from build123d import *

# Parameters (mm, degrees)
F0_W     = 117
F0_H     = 37
F1_DEPTH = 1300
F3_DEPTH = 1300


with BuildPart() as f1:
    # F0 (on Top) → F1 (new body)
    with BuildSketch(Plane.XY):
        with BuildLine():
            ThreePointArc((60, 19.6), (59.882843, 19.882843), (59.6, 20))
            Line((59.6, 20), (-59.6, 20))
            ThreePointArc((-59.6, 20), (-59.882843, 19.882843), (-60, 19.6))
            Line((-60, 19.6), (-60, -19.6))
            ThreePointArc((-60, -19.6), (-59.882843, -19.882843), (-59.6, -20))
            Line((-59.6, -20), (59.6, -20))
            ThreePointArc((59.6, -20), (59.882843, -19.882843), (60, -19.6))
            Line((60, -19.6), (60, 19.6))
        make_face()
        Rectangle(F0_W, F0_H, mode=Mode.SUBTRACT)
    extrude(amount=F1_DEPTH)

    # F2 (on face) → F3 (cut)
    with BuildSketch(Plane.XY.offset(1300)):
        with BuildLine():
            Line((-60, 0), (-58.5, 0))
            Line((-58.5, 0), (-58.5, 18.5))
            Line((-58.5, 18.5), (58.5, 18.5))
            Line((58.5, 18.5), (58.5, 0))
            Line((58.5, 0), (60, 0))
            Line((60, 0), (60, 19.6))
            ThreePointArc((60, 19.6), (59.882843, 19.882843), (59.6, 20))
            Line((59.6, 20), (-59.6, 20))
            ThreePointArc((-59.6, 20), (-59.882843, 19.882843), (-60, 19.6))
            Line((-60, 19.6), (-60, 0))
        make_face()
    extrude(amount=-F3_DEPTH, mode=Mode.SUBTRACT)


solid = f1.part
CAD build for the part. Positions are in the model's coordinates, mm. Round coordinates to 2 decimals unless told otherwise and drop trailing zeros. Loops run counter-clockwise (first coordinate to the right, second up) from the corner with the lowest first, then second, coordinate; pieces in that order, holes last. Notation, with made-up numbers: M 80.25,-24.5 L 107.25,-24.5 A25 ccw 107.25,-1.5 Z; hole C 86,70.5 d8. An arc over 180 degrees is marked long. One line per question, with ' | ' between items. Start each with the question number.
Item 1: Cut at B-B, the plane z = 82. Write the cut outline in (x, y).
Item 2: Two-plate mould, pull along X, no slides. Class faces 1 (the flat face through (-1, -18.5, 641)), 2 (the flat face through (-0.3, -19.6, 1300)), 3 (the flat face through (-60, -10, 641)): pulls with the +X half, pulls with the -X half, needs draft (parallel to the pull), parting line crosses it, or undercut.
Item 3: Wall check: line 1 (X direction, y = -6.5, z = 940); line 2 (Y direction, x = 38, z = 104). Give the ranges that are in metal, low to high.
Item 4: Cut at A-A, the plane y = -13.25. Write the cut outline in (x, z), plus the area to 3 significant figures.
Item 5: Cut at C-C, the plane x = -45.5. Write the cut outline in (y, z).
Item 6: Pin check, flat tip, straight feed: pin 1 Ø12 at (x, z) = (5, 794.5) entering from +Y. Stop position of the tip, or through.
Responses:
1) outline: M -60,-19.6 A0.4 ccw -59.6,-20 L 59.6,-20 A0.4 ccw 60,-19.6 L 60,0 L 58.5,0 L 58.5,-18.5 L -58.5,-18.5 L -58.5,0 L -60,0 Z
2) face 1: undercut | face 2: needs draft | face 3: pulls with the -X half
3) line 1: x = -60 to -58.5, 58.5 to 60 | line 2: y = -20 to -18.5
4) outline: M -60,0 L -58.5,0 L -58.5,1300 L -60,1300 Z; M 58.5,0 L 60,0 L 60,1300 L 58.5,1300 Z | area: 3,900 mm²
5) outline: M -20,0 L -18.5,0 L -18.5,1300 L -20,1300 Z
6) pin 1: stops at y = -18.5
